Build history of the part. All positions in model axes, mm. A direction names the side the tool comes from. Coordinates: 2 decimals unless noted, no trailing zeros. Loops run counter-clockwise (first coordinate to the right, second up) from the corner with the lowest first, then second, coordinate; pieces in that order, holes last.
Item 1: Cut at A-A (z = 6). List the corners of the cut face in (x, y).
Item 2: Cut at C-C (y = -4.75). List the corners of the cut face in (x, z).
Item 3: Drill centre lines: line 1 along X through (y, z) = (3.75, -6.25); line 2 along X through (y, z) = (6.75, 0.25); line 3 along Z through (x, y) = (-2.5, 0). Where is each one in solid material? Low to high.
Item 4: Mould opens along Z. For faces 1 (the face through (-3.986, -2.139, -2.996)), 2 (the face through (0, -7, -1)), 3 (the face through (-2, 0, 7)), 4 (the face through (0, -1, 0)) say: released by +Z, released by -Z, zero draft, split by the parting line, or undercut.
Item 5: Flat gauge pins, fed straight in: pin 1 (1.5 mm diameter, centred on x = 1, y = 2, fed in from +Z); pin 2 (1.7 mm diameter, centred on x = 0.5, z = -7, fed in from +Y); pin 3 (3 mm diameter, centred on x = 2.5, y = 3.5, fed in from -Z). Where does each tip first touch, or does it go through?
Item 6: Cut at D-D (x = 2.75). List the corners of the cut face in (y, z).
Item 7: 3-axis set-ups, long thin cutter, end or side, ignore diameter. For faces 5 (the face through (0, -7, 1)), 6 (the face through (-3, -2, 3)), 7 (the face through (-1, -5, -5)): which of +Z, -Z, +X, -X, +Y, -Y reach the whole face in a straight line?
Item 8: Cut at B-B (x = -3.75). List the corners of the cut face in (y, z).
Autodesk Inventor part; units mm, degrees
ref_plane "YZ Plane" through (0, 0, 0) normal (1, 0, 0) x (0, 1, 0)
ref_plane "XZ Plane" through (0, 0, 0) normal (0, 1, 0) x (-1, 0, 0)
ref_plane "XY Plane" through (0, 0, 0) normal (0, 0, 1) x (1, 0, 0)
sketch "Szkic1" plane through (0, 0, 0) normal (1, 0, 0) x (0, 1, 0)
  circle A0 centre (0, 0) radius 6.5
  circle A1 centre (0, 0) radius 1.75
  line L0 (0, 1.75) -> (0, -1.0846)
  line L1 (-1, 1.9718) -> (-1, -1.0846)
  line L2 (8, 0) -> (-8, 0)
  line L3 (-8, 0) -> (-8, -1)
  line L4 (-8, -1) -> (8, -1)
  line L5 (8, -1) -> (8, 0)
  line L6 (8, 0) -> (-8, 0)
  line L7 (-8, 0) -> (-8, 1)
  line L8 (-8, 1) -> (8, 1)
  line L9 (8, 1) -> (8, 0)
  line L10 (0, 8) -> (1, 8)
  line L11 (1, 8) -> (1, -8)
  line L12 (1, -8) -> (0, -8)
  line L13 (0, 8) -> (-1, 8)
  line L14 (-1, 8) -> (-1, -8)
  line L15 (-1, -8) -> (0, -8)
  line L16 (0, -8) -> (0, 8)
  point P0 (-1, -1.4361)
  point P1 (-1, 1.4361)
  point P2 (-6.4226, -1)
  point P3 (-6.4226, 1)
  point P4 (1, -6.4226)
  point P5 (-1, -6.4226)
  point P6 (6.4226, 1)
  point P7 (6.4226, -1)
  point P8 (-1, 6.4226)
  point P9 (1, 6.4226)
  dimension "d1" = 3.5
  dimension "d0" = 13
  dimension "d2" = 1
  dimension "d14" = 16
  dimension "d16" = 16
  dimension "d18" = 2
  dimension "d19" = 2
sketch "Szkic2" plane through (0, 0, 0) normal (0, 0, 1) x (1, 0, 0)
  line L0 (0, 0) -> (5, 0)
  line L1 (5, 0) -> (5, 6)
  line L2 (5, 6) -> (0, 6)
  line L3 (0, 6) -> (0, 0)
  line L4 (0, 0) -> (-5, 0)
  line L5 (-5, 0) -> (-5, 6)
  line L6 (-5, 6) -> (0, 6)
  line L7 (0, 6) -> (0, 0)
  line L8 (0, 0) -> (5, 0)
  line L9 (5, 0) -> (5, -6)
  line L10 (5, -6) -> (0, -6)
  line L11 (0, -6) -> (0, 0)
  line L12 (0, 0) -> (-5, 0)
  line L13 (-5, 0) -> (-5, -6)
  line L14 (-5, -6) -> (0, -6)
  line L15 (0, -6) -> (0, 0)
  line L16 (5, 6) -> (4, 6)
  line L17 (4, 6) -> (4, 8)
  line L18 (4, 8) -> (5, 8)
  line L19 (5, 8) -> (5, 6)
  line L20 (2, 6) -> (1, 6)
  line L21 (1, 6) -> (1, 8)
  line L22 (1, 8) -> (2, 8)
  line L23 (2, 8) -> (2, 6)
  line L24 (-5, 6) -> (-4, 6)
  line L25 (-4, 6) -> (-4, 8)
  line L26 (-4, 8) -> (-5, 8)
  line L27 (-5, 8) -> (-5, 6)
  line L28 (-2, 6) -> (-1, 6)
  line L29 (-1, 6) -> (-1, 8)
  line L30 (-1, 8) -> (-2, 8)
  line L31 (-2, 8) -> (-2, 6)
  point P0 (-1, 6)
  point P1 (1, 6)
  point P2 (0, 6)
  dimension "d3" = 5
  dimension "d4" = 6
  dimension "d5" = 10
  dimension "d6" = 12
  dimension "d7" = 1
  dimension "d8" = 2
  dimension "d9" = 1
  dimension "d10" = 1
  dimension "d11" = 2
  dimension "d12" = 1
  dimension "d13" = 2
extrude "Wyciągnięcie proste1" add sketch "Szkic1" along normal mid plane 10 contours L2 A1 L8 A0 | A0 L4 A1 L2 | L8 A1 L11 A0 | A0 L11 A1 L4 | L11 A1 L16 A0 | A0 L16 A1 L11 | L16 A1 L1 L14 A0 | A0 L14 A1 L16 | L14 L1 A1 L8 A0 | A0 L4 A1 L14 | L2 A1 L8 L1 | L1 L4 A1 L2 | L8 A1 L2 A0 | L1 L8 A1 | A0 L2 A1 L4 | A1 L4 L1 L14
extrude "Wyciągnięcie proste2" add sketch "Szkic1" along normal mid plane 2 contours L2 L5 L4 A0 | A0 L8 L9 L2 | A0 L16 L10 L11 | L11 L12 L16 A0 | A0 L14 L13 L16 | L16 L15 L14 A0 | A0 L2 L7 L8 | L4 L3 L2 A0
revolve "Obrót1" add sketch "Szkic2" angle 360 about axis through (0, 0, 0) along (1, 0, 0) contours L2 L17 L18 L19 | L21 L22 L23 L2 | L6 L31 L30 L29 | L27 L26 L25 L6
sketch "Sketch3" plane through (-5, 0, 0) normal (-1, 0, 0) x (0, 0, 1)
  circle A0 centre (0, 0) radius 3.5355
  point P0 (2.4008, 2.5954)
  point P1 (-2.5954, 2.4008)
  point P2 (-2.4008, -2.5954)
  point P3 (2.5954, -2.4008)
  dimension "d25" = 7.071
  dimension "d28" = 360
hole "Hole2" at (-5, 2.5954, 2.4008) at (-5, 2.4008, -2.5954) at (-5, -2.5954, -2.4008) at (-5, -2.4008, 2.5954) direction (1, 0, 0) diameter 1.5 depth 2
properties part number "srodek-kolo"
Filled sheet:
1. outline: (-5, -5.29) - (-4, -5.29) - (-4, -2.5) - (-2, -2.5) - (-2, -5.29) - (-1, -5.29) - (-1, -2.5) - (1, -2.5) - (1, -5.29) - (2, -5.29) - (2, -2.5) - (4, -2.5) - (4, -5.29) - (5, -5.29) - (5, 5.29) - (4, 5.29) - (4, 2.5) - (2, 2.5) - (2, 5.29) - (1, 5.29) - (1, 2.5) - (-1, 2.5) - (-1, 5.29) - (-2, 5.29) - (-2, 2.5) - (-4, 2.5) - (-4, 5.29) - (-5, 5.29) - close
2. outline: (-5, -6.44) - (-4, -6.44) - (-4, -4.44) - (-2, -4.44) - (-2, -6.44) - (-1, -6.44) - (-1, -4.44) - (1, -4.44) - (1, -6.44) - (2, -6.44) - (2, -4.44) - (4, -4.44) - (4, -6.44) - (5, -6.44) - (5, 6.44) - (4, 6.44) - (4, 4.44) - (2, 4.44) - (2, 6.44) - (1, 6.44) - (1, 4.44) - (-1, 4.44) - (-1, 6.44) - (-2, 6.44) - (-2, 4.44) - (-4, 4.44) - (-4, 6.44) - (-5, 6.44) - close
3. line 1: x = -5 to -4, -2 to -1, 1 to 2, 4 to 5
3. line 2: x = -5 to -4, -2 to 2, 4 to 5
3. line 3: z = -6.5 to -1.75, 1.75 to 6.5
4. face 1: undercut
4. face 2: released by -Z
4. face 3: zero draft
4. face 4: undercut
5. pin 1: stops at z = 7.9
5. pin 2: stops at y = 4.91
5. pin 3: stops at z = -7.72
6. outline: circle Ø13 at (0, 0); hole (-1, -1.44) arc R1.75 ccw (long way) to (-1, 1.44) - close
7. face 5: +Z, -Y
7. face 6: -X
7. face 7: -Z, -Y
8. outline: circle Ø13 at (0, 0); hole circle Ø1.5 at (-2.6, -2.4); hole circle Ø1.5 at (-2.4, 2.6); hole (-1, -1.44) arc R1.75 ccw (long way) to (-1, 1.44) - close; hole circle Ø1.5 at (2.4, -2.6); hole circle Ø1.5 at (2.6, 2.4)
